The model under review builds one solid part; all positions refer to its coordinate system, in mm. Face numbers are marked on the shaded views. A direction names the side the tool comes from. Coordinates: 2 decimals unless noted, no trailing zeros. Write each loop counter-clockwise with the first axis right and the second up, starting at its lowest first coordinate (ties: lowest second). Pieces come first, ordered by that corner, then holes.
1) Add section C-C, the plane x = 15.75. State the section outline as (y, z) points, then the cut area to 3 significant figures.
2) Add section D-D, the plane z = -6.5. State the section outline as (x, y) points.
3) Mouldability with a two-part tool opening along Z and no side actions: class the marked faces 1, 2 and 3 as released by +Z, released by -Z, zero draft, split by the parting line, or undercut.
4) For P1, Ø3, axis at x = 4.5, y = 6, coming from the -Z side (3 decimals); P2, Ø1.7, axis at x = 4, y = 6, coming from the +Z side (3 decimals), all flat-tipped, find the tip position at first contact; note any pin that passes through.
5) Add section B-B, the plane y = 0.75. State the section outline as (x, z) points.
6) Add section A-A, the plane x = 4.5. State the section outline as (y, z) points (3 decimals), then the cut area to 3 significant figures.
7) Machinability: for the marked faces 4, 5, 6 and 7, which of the approach directions +Z, -Z, +X, -X, +Y, -Y give a long, thin tool a straight path to every point of the face, cutting with its end or side? Answer none if there is none.
8) For line 1 (Z direction, x = 14.51, y = 1.8); line 2 (X direction, y = 0.85, z = -4); line 3 (Y direction, x = 16.25, z = -17.75), list the stretches that pass through material, from the lowest coordinate up.
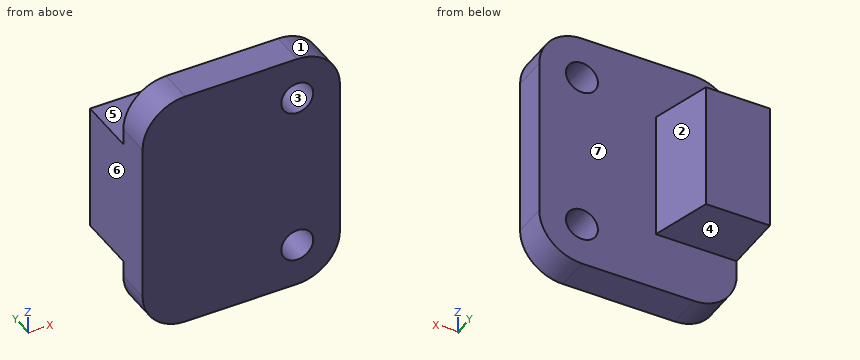
from build123d import *

# Parameters (mm, degrees)
SKETCH1_R           = 1.5
BOSS_EXTRUDE1_DEPTH = 3.22
SKETCH3_W           = 6
SKETCH3_H           = 11.95
BOSS_EXTRUDE2_DEPTH = 5.59
BOSS_EXTRUDE3_DEPTH = 11.95


with BuildPart() as part:
    # Sketch1 → Boss-Extrude1 (new body)
    with BuildSketch(Plane(origin=(0, 0, 0), x_dir=(1, 0, 0), z_dir=(0, 1, 0))):
        with BuildLine():
            Line((4, 0), (14.51, 0))
            ThreePointArc((14.51, 0), (17.338427125, 1.171572875), (18.51, 4))
            Line((18.51, 4), (18.51, 19))
            ThreePointArc((18.51, 19), (17.338427125, 21.828427125), (14.51, 23))
            Line((14.51, 23), (4, 23))
            ThreePointArc((4, 23), (1.171572875, 21.828427125), (0, 19))
            Line((0, 19), (0, 4))
            ThreePointArc((0, 4), (1.171572875, 1.171572875), (4, 0))
        make_face()
        with Locations(Location((14.51, 19, 0), (0, 0, 90))):
            Circle(SKETCH1_R, mode=Mode.SUBTRACT)
        with Locations(Location((14.51, 4, 0), (0, 0, 90))):
            Circle(SKETCH1_R, mode=Mode.SUBTRACT)
    extrude(amount=BOSS_EXTRUDE1_DEPTH)

    # Sketch3 → Boss-Extrude2 (add)
    with BuildSketch(Plane(origin=(0, 3.22, 0), x_dir=(1, 0, 0), z_dir=(0, 1, 0))):
        with Locations((3, 11.5)):
            Rectangle(SKETCH3_W, SKETCH3_H)
    extrude(amount=BOSS_EXTRUDE2_DEPTH)

    # Sketch4 → Boss-Extrude3 (add)
    with BuildSketch(Plane.XY.offset(-5.525)):
        Polygon((0, 3.22), (7.58, 3.22), (6, 8.81), (0, 8.81), align=None)
    extrude(amount=-BOSS_EXTRUDE3_DEPTH)


solid = part.part
Geometry results:
1. outline: (0, -22.8) - (3.22, -22.8) - (3.22, -19.84) - (0, -19.84) - close; (0, -18.16) - (3.22, -18.16) - (3.22, -4.84) - (0, -4.84) - close; (0, -3.16) - (3.22, -3.16) - (3.22, -0.2) - (0, -0.2) - close
1. area: 61.9 mm2
2. outline: (0, 0) - (18.51, 0) - (18.51, 3.22) - (7.58, 3.22) - (6, 8.81) - (0, 8.81) - close
3. face 1: released by +Z
3. face 2: zero draft
3. face 3: undercut
4. P1: stops at z = -17.475
4. P2: stops at z = -5.525
5. outline: (0, -19) arc R4 ccw to (4, -23) - (14.51, -23) arc R4 ccw to (18.51, -19) - (18.51, -4) arc R4 ccw to (14.51, 0) - (4, 0) arc R4 ccw to (0, -4) - close; hole circle Ø3 at (14.51, -19); hole circle Ø3 at (14.51, -4)
6. outline: (0, -23) - (3.22, -23) - (3.22, -17.475) - (8.81, -17.475) - (8.81, -5.525) - (3.22, -5.525) - (3.22, 0) - (0, 0) - close
6. area: 141 mm2
7. face 4: -Z, +X, -X, +Y
7. face 5: +Z, +X, -X, +Y
7. face 6: +Z, -Z, -X, +Y, -Y
7. face 7: +X, +Y
8. line 1: z = -23 to -20.5, -17.5 to -5.5, -2.5 to 0
8. line 2: x = 0 to 13.01, 16.01 to 18.51
8. line 3: y = 0 to 3.22
